Build history of the part. All positions in model axes, mm. Round coordinates to 2 decimals unless told otherwise and drop trailing zeros. Write each loop counter-clockwise with the first axis right and the second up, starting at its lowest first coordinate (ties: lowest second). Pieces come first, ordered by that corner, then holes. Notation, with made-up numbers: (55.5, 18) -> (86.5, 18) arc R35 cw to (86.5, 56) -> close; hole circle Ø11 at (79, 88). An arc over 180 degrees is marked (long way). Return JSON: item names as keys, results as strings.
from build123d import *

# Parameters (mm, degrees)
SKETCH1_W           = 901.7
SKETCH1_H           = 114.3
BOSS_EXTRUDE1_DEPTH = 12.7
SKETCH2_W           = 12.7
SKETCH2_H           = 114.3
CUT_EXTRUDE1_DEPTH  = 6.35
CUT_EXTRUDE2_REACH  = 911.004
SKETCH3_R           = 20.828


with BuildPart() as part:
    # Sketch1 → Boss-Extrude1 (new body)
    with BuildSketch(Plane.XY):
        with Locations((450.85, 57.15)):
            Rectangle(SKETCH1_W, SKETCH1_H)
    extrude(amount=BOSS_EXTRUDE1_DEPTH)

    # Sketch2 → Cut-Extrude1 (cut)
    with BuildSketch(Plane.XY.offset(12.7)):
        with Locations((317.5, 57.15)):
            Rectangle(SKETCH2_W, SKETCH2_H)
        with Locations((584.2, 57.15)):
            Rectangle(SKETCH2_W, SKETCH2_H)
    extrude(amount=-CUT_EXTRUDE1_DEPTH, mode=Mode.SUBTRACT)

    # Sketch3 → Cut-Extrude2 (cut, up to next)
    with BuildSketch(Plane(origin=(0, 0, 0), x_dir=(-1, 0, 0), z_dir=(0, 0, -1)), mode=Mode.PRIVATE) as cut_extrude2_sk1:
        with Locations((-647.7, 38.1)):
            Circle(SKETCH3_R)
    cut_extrude2_tool1 = extrude(cut_extrude2_sk1.sketch, amount=-CUT_EXTRUDE2_REACH, mode=Mode.PRIVATE) & part.part
    # Sketch3 → Cut-Extrude2 (cut, up to next)
    with BuildSketch(Plane(origin=(0, 0, 0), x_dir=(-1, 0, 0), z_dir=(0, 0, -1)), mode=Mode.PRIVATE) as cut_extrude2_sk2:
        with Locations((-254, 38.1)):
            Circle(SKETCH3_R)
    cut_extrude2_tool2 = extrude(cut_extrude2_sk2.sketch, amount=-CUT_EXTRUDE2_REACH, mode=Mode.PRIVATE) & part.part
    add(cut_extrude2_tool1.solids().sort_by_distance((647.7, 38.1, 0))[0], mode=Mode.SUBTRACT)
    add(cut_extrude2_tool2.solids().sort_by_distance((254, 38.1, 0))[0], mode=Mode.SUBTRACT)


solid = part.part
Q1. Saw through at C-C on z = 3. List the corners of the cut face in (x, y).
Verdict:
{"outline": "(0, 0) -> (901.7, 0) -> (901.7, 114.3) -> (0, 114.3) -> close; hole circle Ø41.66 at (254, 38.1); hole circle Ø41.66 at (647.7, 38.1)"}
Q2. Wall check: L1, parallel to X at y = 10, z = 9; L2, parallel to X at y = 40, z = 4; L3, parallel to Y at x = 647.7, z = 3.25. Give the ranges that are in metal, low to high.
Verdict:
{"L1": "x = 0 to 311.15, 323.85 to 577.85, 590.55 to 901.7", "L2": "x = 0 to 233.26, 274.74 to 626.96, 668.44 to 901.7", "L3": "y = 0 to 17.27, 58.93 to 114.3"}
Q3. Pin check, flat tip, straight feed: pin 1 Ø4 at (x, y) = (315.5, 29.5) entering from +Z. Stop position of the tip, or through.
Verdict:
{"pin 1": "stops at z = 6.35"}
Q4. Saw through at A-A on y = 38.1. List the corners of the cut face in (x, z).
Verdict:
{"outline": "(0, 0) -> (233.17, 0) -> (233.17, 12.7) -> (0, 12.7) -> close; (274.83, 0) -> (626.87, 0) -> (626.87, 12.7) -> (590.55, 12.7) -> (590.55, 6.35) -> (577.85, 6.35) -> (577.85, 12.7) -> (323.85, 12.7) -> (323.85, 6.35) -> (311.15, 6.35) -> (311.15, 12.7) -> (274.83, 12.7) -> close; (668.53, 0) -> (901.7, 0) -> (901.7, 12.7) -> (668.53, 12.7) -> close"}
Q5. Two-plate mould, pull along Y, no slides. Class faces 1 (the flat face through (449, 58, 12.7)), 2 (the cylindrical face through (234.134, 44.356, 6.261)): +Y half, -Y half, draft (parallel to the pull), parting line (faces both ways), or undercut.
Verdict:
{"face 1": "draft", "face 2": "undercut"}
Q6. Saw through at B-B on x = 647.7. List the corners of the cut face in (y, z).
Verdict:
{"outline": "(0, 0) -> (17.27, 0) -> (17.27, 12.7) -> (0, 12.7) -> close; (58.93, 0) -> (114.3, 0) -> (114.3, 12.7) -> (58.93, 12.7) -> close"}
